from build123d import *

# Parameters (mm, degrees)
F1_DEPTH = 88.9
F2_R     = 0.99999


# Not quite as in the source:
# - a fillet or chamfer is up to 0.001 mm smaller than in the source, because OpenCascade refuses the exact size


with BuildPart() as f1:
    # F0 (on Right) → F1 (new body, symmetric)
    with BuildSketch(Plane.YZ):
        Polygon((0, 17.78), (0, 0), (12.7, 0), (12.7, 2), (2, 2), (2, 17.78), align=None)
    extrude(amount=F1_DEPTH, both=True)

    # F2 (radius 1 in the source; OpenCascade refuses exactly that, so slightly less here)
    f2_edges = [f1.edges().sort_by_distance(p)[0] for p in [
        (0, 0, 17.78),
        (88.9, 0, 8.89),
        (-88.9, 1, 17.78),
        (88.9, 1, 17.78),
        (0, 2, 17.78),
        (88.9, 2, 9.89),
        (88.9, 6.35, 0),
        (88.9, 12.7, 1),
        (88.9, 7.35, 2),
        (-88.9, 0, 8.89),
        (-88.9, 2, 9.89),
        (-88.9, 7.35, 2),
        (-88.9, 6.35, 0),
    ]]
    fillet(f2_edges, radius=F2_R)


solid = f1.part
Work out the finished part from the listing and answer in its coordinate system (mm). A direction names the side the tool comes from. Give positions to 0.01 mm unless a question says otherwise; leave off trailing zeros. Answer in a Markdown table with one row per item.
(1) Flat-ended cylindrical pins translate along their axes: pin 1 Ø4 at (x, y) = (8.5, 11.5) entering from +Z; pin 2 Ø7.5 at (x, z) = (-5.5, 11.5) entering from +Y; pin 3 Ø1.5 at (x, y) = (-32.5, 2) entering from +Z. Find the tip coordinate at first contact, or state that the pin passes through.
Results list:
| item | result |
|---|---|
| pin 1 | stops at z = 2 |
| pin 2 | stops at y = 2 |
| pin 3 | stops at z = 17.75 |
(2) Consider L1, parallel to Y at x = 44, z = 11.5; L2, parallel to X at y = 1.5, z = 1.5. Determine where each line is inside the solid, lowest interval first. Write a range as [from, to].
Results list:
| item | result |
|---|---|
| L1 | y = [0, 2] |
| L2 | x = [-88.77, 88.77] |
(3) A tool of negligible diameter and unlimited length cuts with its end or side. For faces 1 (the face through (1, 7, 2)), 2 (the face through (1, 6, 0)), from which of +Z, -Z, +X, -X, +Y, -Y can it reach the whole face along a straight path? Write none if from no direction.
Results list:
| item | result |
|---|---|
| face 1 | +Z, +X, -X, +Y |
| face 2 | -Z, +X, -X, +Y, -Y |
